The listing builds one solid part. Answer for the finished solid, in the listing's coordinates (mm). A direction names the side the tool comes from. Give positions to 0.01 mm unless a question says otherwise; leave off trailing zeros. Order: outer loops, then holes, each group sorted by start corner. A loop starts at its lowest first (then second) coordinate and runs counter-clockwise, first axis right, second up. Notation, with made-up numbers: (72.25, 38) - (101.25, 38) arc R19 cw to (101.25, 69) - close; hole circle Ø4 at (51, 20.5). An arc over 180 degrees is marked (long way). Answer in a Markdown table with one row per item. Add a question column.
```python
from build123d import *

# Parameters (mm, degrees)
F0_R      = 60
F1_DEPTH  = 25
F2_R      = 11
F4_DEPTH  = 9
F3_R      = 45
F3_R_2    = 11
F5_DEPTH  = 0.01
F6_DEPTH  = 2
F7_R      = 11
F9_DEPTH  = 9
F8_R      = 45
F10_DEPTH = 2
F11_R     = 12.5
F12_R     = 12.49999
F13_R     = 8.5
F14_DEPTH = 25


# Not quite as in the source:
# - a fillet or chamfer is up to 0.001 mm smaller than in the source, because OpenCascade refuses the exact size


with BuildPart() as f1:
    # F0 (on Top) → F1 (new body)
    with BuildSketch(Plane.XY):
        Circle(F0_R)
    extrude(amount=F1_DEPTH)

    # F2 (on face) → F4 (cut)
    with BuildSketch(Plane.XY.offset(25)):
        Circle(F2_R)
    extrude(amount=-F4_DEPTH, mode=Mode.SUBTRACT)

    # F3 (on face) → F5 (cut)
    with BuildSketch(Plane.XY.offset(25)):
        Circle(F3_R)
        Circle(F3_R_2, mode=Mode.SUBTRACT)
    extrude(amount=-F5_DEPTH, mode=Mode.SUBTRACT)

    # F3 (on face) → F6 (cut)
    with BuildSketch(Plane.XY.offset(25)):
        Circle(F3_R)
    extrude(amount=-F6_DEPTH, mode=Mode.SUBTRACT)

    # F7 (on face) → F9 (cut)
    with BuildSketch(Plane(origin=(0, 0, 0), x_dir=(1, 0, 0), z_dir=(0, 0, -1))):
        Circle(F7_R)
    extrude(amount=-F9_DEPTH, mode=Mode.SUBTRACT)

    # F8 (on face) → F10 (cut)
    with BuildSketch(Plane(origin=(0, 0, 0), x_dir=(1, 0, 0), z_dir=(0, 0, -1))):
        Circle(F8_R)
    extrude(amount=-F10_DEPTH, mode=Mode.SUBTRACT)

    # F11
    f11_edges = [f1.edges().sort_by_distance(p)[0] for p in [
        (-60, 0, 25),
    ]]
    fillet(f11_edges, radius=F11_R)

    # F12 (radius 12.5 in the source; OpenCascade refuses exactly that, so slightly less here)
    f12_edges = [f1.edges().sort_by_distance(p)[0] for p in [
        (-60, 0, 0),
    ]]
    fillet(f12_edges, radius=F12_R)

    # F13 (on face) → F14 (cut)
    with BuildSketch(Plane.XY.offset(16)):
        Circle(F13_R)
    extrude(amount=-F14_DEPTH, mode=Mode.SUBTRACT)


solid = f1.part
```
(1) Each of these flat-tipped pins is pushed along its axis until it touches: P1, Ø1, axis at y = -43.5, z = 21.5, coming from the -X side; P2, Ø13, axis at x = 0, y = 0, coming from the +Z side; P3, Ø24, axis at x = -2.5, y = 5.5, coming from the -Z side; P4, Ø12, axis at x = -26, z = 5, coming from the +Y side. Where does it stop, or does it pass through?
(2) Find section C-C, the plane z = 10.5. Write down the section's boundary in (x, y).
(3) Straight lines are drawn through the part: line 1 (Y direction, x = 0, z = 24); line 2 (X direction, y = 4, z = 17.5); line 3 (Y direction, x = 0, z = 14). For each, find the intervals that lie inside material, in ascending order.
(4) The mould has two halves that part along X. Classify faces 1 (the face through (42, -17, 0)), 2 (the face through (9, 9, 2)): +X half, -X half, draft (parallel to the pull), parting line (faces both ways), or undercut.
(5) For faces 3 (the face through (9, -9, 23)), 4 (the face through (3.2, 8.1, 9)), 5 (the face through (42, -17, 25)), determine the directions among +Z, -Z, +X, -X, +Y, -Y from which every point of the face is accessible in a straight line to the end or side of a thin tool.
Answer key:
| question | item | result |
|---|---|---|
| 1 | P1 | x = -36.53 |
| 1 | P2 | through |
| 1 | P3 | z = 2 |
| 1 | P4 | y = 55.47 |
| 2 | outline | circle Ø119.68 at (0, 0); hole circle Ø17 at (0, 0) |
| 3 | line 1 | -52.4 to -45, 45 to 52.4 |
| 3 | line 2 | -58.82 to -10.25, 10.25 to 58.82 |
| 3 | line 3 | -59.91 to -8.5, 8.5 to 59.91 |
| 4 | face 1 | draft |
| 4 | face 2 | undercut |
| 5 | face 3 | +Z |
| 5 | face 4 | -Z |
| 5 | face 5 | +Z, +X, -X, +Y, -Y |
